Autodesk Inventor part; units mm, degrees
ref_plane "IP1_XY" through (0, 0, 0) normal (1, 0, 0) x (0, 0, -1)
ref_plane "IP1_YZ" through (0, 0, 0) normal (0, 0, -1) x (0, 1, 0)
ref_plane "IP1_ZX" through (0, 0, 0) normal (0, 1, 0) x (1, 0, 0)
sketch "Skizze_2" plane through (-3.1, 0, 0) normal (1, 0, 0) x (0, 0, -1)
  arc A0 (-1.6711, 0.3843) -> (-1.6711, -0.3843) centre (-1.58, 0) ccw
  arc A1 (-1.1684, -1.2551) -> (-1.6711, -0.3843) centre (-1.8307, -1.0569) ccw
  arc A2 (-1.1684, -1.2551) -> (-0.5027, -1.6394) centre (-0.79, -1.3683) ccw
  arc A3 (0.5027, -1.6394) -> (-0.5027, -1.6394) centre (0, -2.1139) ccw
  arc A4 (0.5027, -1.6394) -> (1.1684, -1.2551) centre (0.79, -1.3683) ccw
  arc A5 (1.6711, -0.3843) -> (1.1684, -1.2551) centre (1.8307, -1.0569) ccw
  arc A6 (1.6711, -0.3843) -> (1.6711, 0.3843) centre (1.58, 0) ccw
  arc A7 (1.1684, 1.2551) -> (1.6711, 0.3843) centre (1.8307, 1.0569) ccw
  arc A8 (1.1684, 1.2551) -> (0.5027, 1.6394) centre (0.79, 1.3683) ccw
  arc A9 (-0.5027, 1.6394) -> (0.5027, 1.6394) centre (0, 2.1139) ccw
  arc A10 (-0.5027, 1.6394) -> (-1.1684, 1.2551) centre (-0.79, 1.3683) ccw
  arc A11 (-1.6711, 0.3843) -> (-1.1684, 1.2551) centre (-1.8307, 1.0569) ccw
sketch "Skizze_3" plane through (0, 0, 0) normal (0, 0, 1) x (1, 0, 0)
  line L0 (-0.1, 0) -> (-0.2997, 0)
  line L1 (-0.2997, 0) -> (-1.4977, 2.075)
  line L2 (-1.4977, 2.075) -> (-0.1, 2.075)
  line L3 (-0.1, 2.075) -> (-0.1, 0)
  line L4 (-0.1, 0) -> (-0.2997, 0)
sketch "Skizze_5" plane through (0, 0, 0) normal (0, 0, 1) x (1, 0, 0)
  line L0 (16, 0) -> (-3.1, 0)
  line L1 (-3.1, 0) -> (-3.1, 3.2288)
  line L2 (-3.1, 3.2288) -> (0, 3.5)
  line L3 (0, 3.5) -> (0, 1.7853)
  line L4 (0, 1.7853) -> (1.028, 1.7853)
  line L5 (1.028, 1.7853) -> (1.4, 2)
  line L6 (1.4, 2) -> (16, 2)
  line L7 (16, 2) -> (16, 0)
  line L8 (16, 0) -> (-3.1, 0)
revolve "Revolution1" add sketch "Skizze_5" angle 360 about axis through (16, 0, 0) along (1, 0, 0)
thread "Thread1"
sketch "Sketch_1" plane through (0, 0, 0) normal (0, 0, 1) x (1, 0, 0)
  line L0 (0.2, 0) -> (-0.1, 0)
  line L1 (-0.1, 1.6853) -> (0.2, 1.6853)
  line L2 (0.2, 1.6853) -> (0.2, 1.7853)
  arc A0 (0, 1.9852) -> (0.2, 1.7853) centre (0.2, 1.9853) ccw
  line L3 (0, 1.9852) -> (-0.1, 1.9852)
  line L4 (-0.1, 1.9852) -> (-0.1, 1.6853)
revolve "Revolution2" add sketch "Sketch_1" angle 360 about axis through (0.2, 0, 0) along (1, 0, 0)
sketch "Sketch_2" plane through (0, 0, 0) normal (0, 0, 1) x (1, 0, 0)
  line L0 (-1.9597, 0) -> (-3.1, 0)
  line L1 (-3.1, 0) -> (-3.1, 1.975)
  line L2 (-3.1, 1.975) -> (-1.9597, 0)
  line L3 (-1.9597, 0) -> (-3.1, 0)
revolve "Revolution3" cut sketch "Sketch_2" angle 360 about axis through (-1.9597, 0, 0) along (1, 0, 0)
sketch "Sketch_3" plane through (0, 0, 0) normal (0, 0, 1) x (1, 0, 0)
  line L0 (50, 0) -> (-3.1, 0)
  line L1 (-3.6, 8.4) -> (-3.6, 2.9081)
  line L2 (-3.6, 2.9081) -> (-3.1, 2.9081)
  arc A0 (-2.7805, 3.2567) -> (-3.1, 2.9081) centre (-2.75, 2.9081) ccw
  line L3 (-2.7805, 3.2567) -> (-2.7805, 8.4)
  line L4 (-2.7805, 8.4) -> (-3.6, 8.4)
revolve "Revolution4" cut sketch "Sketch_3" angle 360 about axis through (50, 0, 0) along (1, 0, 0)
extrude "Extrusion1" cut sketch "Skizze_2" along normal blind 2.79
revolve "Revolution5" add sketch "Skizze_3" angle 360 about axis through (-0.1, 0, 0) along (1, 0, 0)
ref_plane "IP1_XY" through (0, 0, 0) normal (1, 0, 0) x (0, 0, -1)
ref_plane "IP1_YZ" through (0, 0, 0) normal (0, 0, -1) x (0, 1, 0)
ref_plane "IP1_ZX" through (0, 0, 0) normal (0, 1, 0) x (1, 0, 0)
properties part number "ISO 14580 M4x16"
Model file for the job. Use its own axes, mm. A direction names the side the tool comes from. Give positions to 0.01 mm unless a question says otherwise; leave off trailing zeros. Order: outer loops, then holes, each group sorted by start corner. A loop starts at its lowest first (then second) coordinate and runs counter-clockwise, first axis right, second up. Notation, with made-up numbers: (7, 63.25) - (56, 63.25) arc R20 cw to (56, 86.25) - close; hole circle Ø10 at (-18.75, -13.75). An arc over 180 degrees is marked (long way). Return JSON: item names as keys, results as strings.
1) Probe line 1 (Y direction, x = 14.25, z = 0.25); line 2 (X direction, y = 1, z = -1); line 3 (X direction, y = 2.75, z = -0.5). List the from-to ranges inside material, lowest first. Write a range as from..to.
Geometry says:
{"line 1": "-1.98..1.98", "line 2": "-1.12..16", "line 3": "-3.1..0"}
2) Pull direction X, two halves, no side cores. Call faces 4 (the cylindrical face through (0.62, -0.387, -1.743)), 5 (the flat face through (16, 0, 0)), 6 (the conical face through (-2.87, 0.82, -1.35)): pulls with the +X half, pulls with the -X half, needs draft (parallel to the pull), parting line crosses it, or undercut.
Geometry says:
{"face 4": "undercut", "face 5": "pulls with the +X half", "face 6": "pulls with the -X half"}
3) 3-axis set-ups, long thin cutter, end or side, ignore diameter. For faces 1 (the flat face through (-3.1, 1, -2)), 2 (the cylindrical face through (-2.05, -0.7, 1.24)), 3 (the cylindrical face through (9, 0, -2)): which of +Z, -Z, +X, -X, +Y, -Y reach the whole face in a straight line?
Geometry says:
{"face 1": "+Z, -Z, -X, +Y, -Y", "face 2": "-X", "face 3": "+X"}
4) Flat gauge pins, fed straight in: P1, Ø2, axis at y = -1.5, z = 2, coming from the +X side; P2, Ø4, axis at x = 4.5, z = 2, coming from the -Y side. Where does each tip first touch, or does it go through?
Geometry says:
{"P1": "x = 16", "P2": "y = -2"}
5) Cut at A-A, the plane x = 10.25. Give the cut face in (y, z), plus the area to 3 significant figures.
Geometry says:
{"outline": "circle Ø4 at (0, 0)", "area": "12.6 mm²"}
